Autodesk Inventor part; units mm, degrees
ref_plane "YZ Plane" through (0, 0, 0) normal (1, 0, 0) x (0, 1, 0)
ref_plane "XZ Plane" through (0, 0, 0) normal (0, 1, 0) x (-1, 0, 0)
ref_plane "XY Plane" through (0, 0, 0) normal (0, 0, 1) x (1, 0, 0)
sketch "Sketch1" plane through (0, 0, 0) normal (0, 1, 0) x (-1, 0, 0)
  line L0 (0, 0) -> (0, 53.3)
  line L1 (0, 53.3) -> (68.5346, 53.3)
  line L2 (68.5346, 53.3) -> (68.5346, 0)
  line L3 (68.5346, 0) -> (0, 0)
  line L4 (68.5346, 0) -> (68.5346, 2.5)
  line L5 (68.5346, 2.5) -> (68.5346, 7.6)
  line L6 (68.5346, 7.6) -> (68.5346, 35.5)
  line L7 (0, 53.3) -> (14, 53.3)
  line L8 (68.5346, 35.5) -> (68.5346, 50.7)
  circle A0 centre (13.5, 50.7) radius 1.4
  circle A1 centre (13.5, 2.5) radius 1.4
  circle A2 centre (64.8, 35.5) radius 1.4
  circle A3 centre (64.8, 7.6) radius 1.4
  line L9 (0, 63.3) -> (78.5346, 63.3)
  line L10 (78.5346, 63.3) -> (78.5346, 0)
  line L11 (-10, 53.3) -> (-10, -10)
  line L12 (-10, -10) -> (68.5346, -10)
  line L13 (-10, -10) -> (78.5346, -10)
  line L14 (78.5346, -10) -> (78.5346, 63.3)
  line L15 (78.5346, 63.3) -> (-10, 63.3)
  line L16 (-10, 63.3) -> (-10, -10)
  line L17 (74.5346, 63.3) -> (74.5346, -6)
  line L18 (74.5346, -6) -> (-10, -6)
  line L19 (78.5346, 59.3) -> (-6, 59.3)
  line L20 (-6, 59.3) -> (-6, -10)
  line L21 (14.5, 50.7) -> (14.5, 2.5)
  dimension "d0" = 53.3
  dimension "d1" = 68.5346
  dimension "d2" = 2.8
  dimension "d3" = 2.8
  dimension "d4" = 2.8
  dimension "d5" = 2.8
  dimension "d6" = 10
  dimension "d7" = 10
  dimension "d8" = 4
  dimension "d9" = 4
  dimension "d10" = 1
  dimension "d11" = 1
extrude "Extrusion1" add sketch "Sketch1" along normal blind 1.5 contours L0 L1 L2 L3 | L9 L17 L19 L20 L18 L11 L16 L15 | L9 L10 L19 L17 | L19 L10 L14 L13 L12 L20 L18 L17 | L17 L18 L20 L19 | L18 L20 L12 L11
sketch "Sketch3" plane through (0, 1.5, 0) normal (0, 1, 0) x (1, 0, 0)
  line L0 (10, -63.3) -> (10, 10)
  line L1 (10, 10) -> (-78.5346, 10)
  line L2 (-78.5346, 10) -> (-78.5346, 21)
  line L3 (-78.5346, 21) -> (10, 21)
  line L4 (10, 21) -> (10, 10)
  line L5 (10, 21) -> (4.5, 21)
  line L6 (4.5, 21) -> (4.5, 15.5)
  line L7 (4.5, 15.5) -> (10, 15.5)
  line L8 (10, 15.5) -> (10, 21)
  circle A0 centre (4.5, 15.5) radius 0.8
  point P0 (0, 0)
  dimension "d14" = 11
  dimension "d15" = 5.5
  dimension "d16" = 5.5
  dimension "d17" = 1.6
extrude "Extrusion2" add sketch "Sketch3" against normal blind 1.5 contours L1 L2 L3 L6 A0 L7 L4 | L7 A0 L6 L3 L4
sketch "Sketch4" plane through (0, 1.5, 0) normal (0, 1, 0) x (1, 0, 0)
  circle A0 centre (4.5, 15.5) radius 0.8
  line L0 (8.7, 15.5) -> (8.7, 20.5)
  line L1 (8.7, 20.5) -> (-11.3, 20.5)
  line L2 (-11.3, 20.5) -> (-11.3, 10.5)
  line L3 (-11.3, 10.5) -> (8.7, 10.5)
  line L4 (8.7, 10.5) -> (8.7, 15.5)
  line L5 (-11.3, 10.5) -> (-11.3, 20.5)
  line L6 (-10.3, 20.5) -> (-10.3, 10.5)
  line L7 (-6.3, 20.5) -> (-6.3, 10.5)
  line L8 (-7.3, 20.5) -> (-7.3, 10.5)
  point P0 (0, 0)
  dimension "d21" = 5
  dimension "d22" = 20
  dimension "d23" = 10
  dimension "d24" = 1
  dimension "d25" = 4
  dimension "d26" = 1
extrude "Extrusion3" cut sketch "Sketch4" against normal blind 15.4 contours L8 L3 L6 L1
properties part number "FitmentCard"
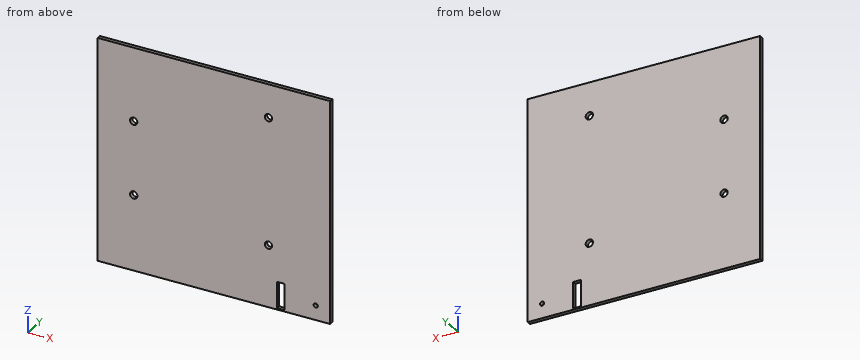
Can you work these out from the model? Positions are in its coordinate system, mm. Coordinates: 2 decimals unless noted, no trailing zeros. Write each loop counter-clockwise with the first axis right and the second up, starting at its lowest first coordinate (ties: lowest second). Pieces come first, ordered by that corner, then holes. Notation, with made-up numbers: M -12,85 L 23,85 A19 cw 23,108 Z; hole C 0.25,-36.5 d3. An arc over 180 degrees is marked long. Use one line per item in the form item = value.
Q1. I need wall thicknesses on line 1 along Z through (x, y) = (-64.8, 0.85); line 2 along X through (y, z) = (0.65, -15.5); line 3 along Z through (x, y) = (-13.5, 0.4). Which ranges of each line are inside material? Lowest first, please. Write a range as from..to.
Model answer:
line_1 = -21..6.2, 9..34.1, 36.9..63.3
line_2 = -78.53..-10.3, -7.3..3.7, 5.3..10
line_3 = -21..1.1, 3.9..49.3, 52.1..63.3
Q2. If we section it at A-A (x = -13.5): Write out the boundary of the cut face in (y, z), then the cut area to 3 significant figures.
Model answer:
outline = M 0,-21 L 1.5,-21 L 1.5,1.1 L 0,1.1 Z; M 0,3.9 L 1.5,3.9 L 1.5,49.3 L 0,49.3 Z; M 0,52.1 L 1.5,52.1 L 1.5,63.3 L 0,63.3 Z
area = 118 mm^2
Q3. If we section it at B-B (z = 50.7): Write out the boundary of the cut face in (x, y).
Model answer:
outline = M -78.53,0 L -14.9,0 L -14.9,1.5 L -78.53,1.5 Z; M -12.1,0 L 10,0 L 10,1.5 L -12.1,1.5 Z
